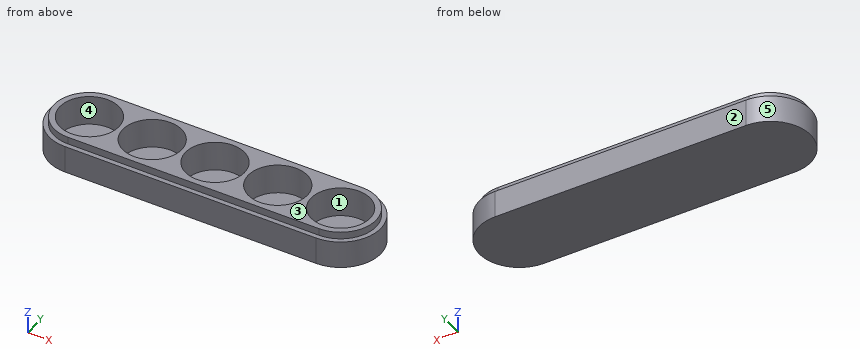
from build123d import *

# Parameters (mm, degrees)
F1_DEPTH = 11.5
F3_DEPTH = 3
F4_R     = 12.5
F5_DEPTH = 12.5


with BuildPart() as f1:
    # F0 (on Top) → F1 (new body)
    with BuildSketch(Plane.XY):
        with BuildLine():
            Line((52.032723, 18.360732), (-55.967277, 18.360732))
            ThreePointArc((-55.967277, 18.360732), (-72.967277, 1.360732), (-55.967277, -15.639268))
            Line((-55.967277, -15.639268), (52.032723, -15.639268))
            ThreePointArc((52.032723, -15.639268), (69.032723, 1.360732), (52.032723, 18.360732))
        make_face()
    extrude(amount=F1_DEPTH)

    # F2 (on face) → F3 (join)
    with BuildSketch(Plane.XY.offset(11.5)):
        with BuildLine():
            ThreePointArc((52.032723, -13.639268), (67.032723, 1.360732), (52.032723, 16.360732))
            Line((52.032723, 16.360732), (-55.967277, 16.360732))
            ThreePointArc((-55.967277, 16.360732), (-70.967277, 1.360732), (-55.967277, -13.639268))
            Line((-55.967277, -13.639268), (52.032723, -13.639268))
        make_face()
    extrude(amount=F3_DEPTH)

    # F4 (on face) → F5 (cut)
    with BuildSketch(Plane.XY.offset(14.5)):
        with Locations((-55.967277, 1.360732)):
            Circle(F4_R)
        with Locations((-28.967277, 1.360732)):
            Circle(F4_R)
        with Locations((-1.967277, 1.360732)):
            Circle(F4_R)
        with Locations((25.032723, 1.360732)):
            Circle(F4_R)
        with Locations((52.032723, 1.360732)):
            Circle(F4_R)
    extrude(amount=-F5_DEPTH, mode=Mode.SUBTRACT)


solid = f1.part
Work out the finished part from the listing and answer in its coordinate system (mm). Face numbers are marked on the shaded views. A direction names the side the tool comes from. Round coordinates to 2 decimals unless told otherwise and drop trailing zeros. Write each loop counter-clockwise with the first axis right and the second up, starting at its lowest first coordinate (ties: lowest second). Pieces come first, ordered by that corner, then holes. Notation, with made-up numbers: (-39.5, 44.5) -> (-19.5, 44.5) arc R36 cw to (-19.5, 82.5) -> close; hole circle Ø4 at (82, -3). An arc over 180 degrees is marked (long way). Write each question's results on one line, items separated by ' | '.
Item 1: Flat-ended cylindrical pins translate along their axes: P1, Ø12.5, axis at x = -61.5, y = -1, coming from the +Z side; P2, Ø20, axis at x = -23.5, y = -1, coming from the +Z side; P3, Ø1.5, axis at x = 24.5, z = 13, coming from the -Y side; P4, Ø5, axis at y = -10.5, z = 4.5, coming from the +X side. Find the tip coordinate at first contact, or state that the pin passes through.
Result set:
P1: z = 2 | P2: z = 14.5 | P3: y = -13.64 | P4: x = 66.22
Item 2: The mould has two halves that part along X. Classify the marked faces 3, 4 and 5: +X half, -X half, draft (parallel to the pull), parting line (faces both ways), or undercut.
Result set:
face 3: draft | face 4: undercut | face 5: -X half
Item 3: A cutting plane is placed at B-B, the plane x = -23. Determine the outline of the cut face in (y, z).
Result set:
outline: (-15.64, 0) -> (18.36, 0) -> (18.36, 11.5) -> (16.36, 11.5) -> (16.36, 14.5) -> (12.34, 14.5) -> (12.34, 2) -> (-9.62, 2) -> (-9.62, 14.5) -> (-13.64, 14.5) -> (-13.64, 11.5) -> (-15.64, 11.5) -> close
Item 4: A cutting plane is placed at D-D, the plane x = -6.5. Determine the outline of the cut face in (y, z).
Result set:
outline: (-15.64, 0) -> (18.36, 0) -> (18.36, 11.5) -> (16.36, 11.5) -> (16.36, 14.5) -> (13.01, 14.5) -> (13.01, 2) -> (-10.29, 2) -> (-10.29, 14.5) -> (-13.64, 14.5) -> (-13.64, 11.5) -> (-15.64, 11.5) -> close
Item 5: A cutting plane is placed at C-C, the plane y = -4.5. Determine the outline of the cut face in (x, z).
Result set:
outline: (-71.93, 0) -> (67.99, 0) -> (67.99, 11.5) -> (65.84, 11.5) -> (65.84, 14.5) -> (63.07, 14.5) -> (63.07, 2) -> (40.99, 2) -> (40.99, 14.5) -> (36.07, 14.5) -> (36.07, 2) -> (13.99, 2) -> (13.99, 14.5) -> (9.07, 14.5) -> (9.07, 2) -> (-13.01, 2) -> (-13.01, 14.5) -> (-17.93, 14.5) -> (-17.93, 2) -> (-40.01, 2) -> (-40.01, 14.5) -> (-44.93, 14.5) -> (-44.93, 2) -> (-67.01, 2) -> (-67.01, 14.5) -> (-69.77, 14.5) -> (-69.77, 11.5) -> (-71.93, 11.5) -> close
Item 6: Which of the six approach directions +Z, -Z, +X, -X, +Y, -Y give full straight-line access (tool end or side, diameter ignored) to the marked faces 1 and 2?
Result set:
face 1: +Z | face 2: +Z, -Z, +X, -X, +Y
Item 7: A cutting plane is placed at A-A, the plane z = 9.75. Determine the outline of the cut face in (x, y), plus the area to 3 significant figures.
Result set:
outline: (-55.97, -15.64) -> (52.03, -15.64) arc R17 ccw to (52.03, 18.36) -> (-55.97, 18.36) arc R17 ccw to start; hole circle Ø25 at (-55.97, 1.36); hole circle Ø25 at (-28.97, 1.36); hole circle Ø25 at (-1.97, 1.36); hole circle Ø25 at (25.03, 1.36); hole circle Ø25 at (52.03, 1.36) | area: 2,130 mm^2
Item 8: Find the intervals of material crossed by line 1 along X through (y, z) = (-1, 6.5); line 2 along Y through (x, z) = (-29, 11.75); line 3 along X through (y, z) = (8.5, 11), in increasing order. Write a range as [from, to].
Result set:
line 1: [-72.8, -68.24], [-43.69, -41.24], [-16.69, -14.24], [10.31, 12.76], [37.31, 39.76], [64.31, 68.87] | line 2: [-13.64, -11.14], [13.86, 16.36] | line 3: [-71.4, -66.23], [-45.71, -39.23], [-18.71, -12.23], [8.29, 14.77], [35.29, 41.77], [62.29, 67.46]
